The drawing under review shows one solid part. Ordinate dimensions are in mm from its lowest x, y, z. Coordinates: 2 decimals unless noted, no trailing zeros. Write each loop counter-clockwise with the first axis right and the second up, starting at its lowest first coordinate (ties: lowest second). Pieces come first, ordered by that corner, then holes. Notation, with made-up numbers: (26.5, 65) -> (45.5, 65) arc R21 ccw to (45.5, 81) -> close; hole circle Ø10 at (36, -18.75). An arc over 180 degrees is marked (long way). One line per question, with ' | ' between items. Start each with the question number.
Q1. Add section D-D on x = 3.5. State the section outline as (y, z) points, and give its area (3 significant figures).
Q2. Add section B-B on y = 1.8. State the section outline as (x, z) points, and give its area (3 significant figures).
Q3. Add section C-C on z = 61.5. State the section outline as (x, y) points, and give its area (3 significant figures).
Q4. Add section A-A on x = 26.5. State the section outline as (y, z) points, and give its area (3 significant figures).
Q5. Wall thickness on probe 1 along Z at (x, y) = (26.5, 1.9); probe 2 along Z at (x, y) = (3.5, 0.85); probe 3 along Z at (x, y) = (27, 2.1): over which ranges is each line inside the solid? List them lowest first.
Q6. For P1, Ø0.9, axis at y = 2, z = 24.5, coming from the +X side, flat-tipped, find the tip position at first contact; note if it passes through.
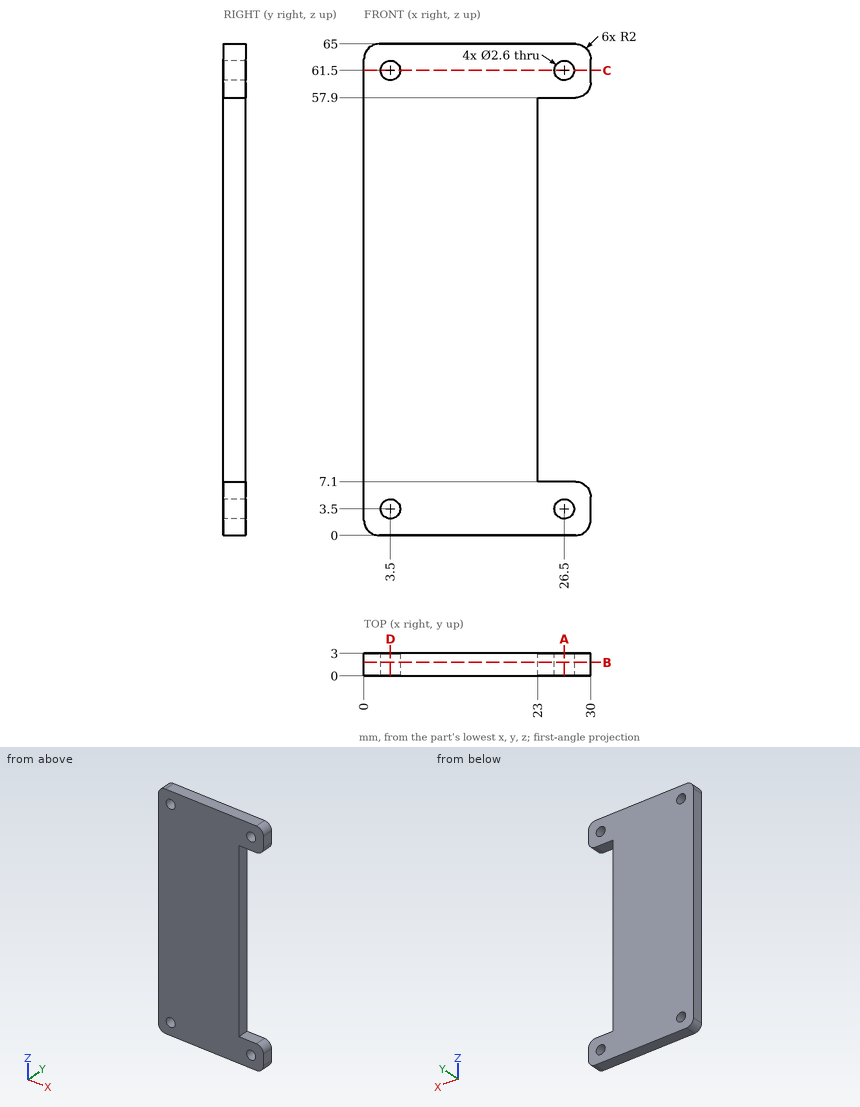
Output values:
1) outline: (0, 0) -> (3, 0) -> (3, 2.2) -> (0, 2.2) -> close; (0, 4.8) -> (3, 4.8) -> (3, 60.2) -> (0, 60.2) -> close; (0, 62.8) -> (3, 62.8) -> (3, 65) -> (0, 65) -> close | area: 179 mm2
2) outline: (0, 2) arc R2 ccw to (2, 0) -> (28, 0) arc R2 ccw to (30, 2) -> (30, 5.1) arc R2 ccw to (28, 7.1) -> (23, 7.1) -> (23, 57.9) -> (28, 57.9) arc R2 ccw to (30, 59.9) -> (30, 63) arc R2 ccw to (28, 65) -> (2, 65) arc R2 ccw to (0, 63) -> close; hole circle Ø2.6 at (3.5, 3.5); hole circle Ø2.6 at (3.5, 61.5); hole circle Ø2.6 at (26.5, 3.5); hole circle Ø2.6 at (26.5, 61.5) | area: 1,570 mm2
3) outline: (0, 0) -> (2.2, 0) -> (2.2, 3) -> (0, 3) -> close; (4.8, 0) -> (25.2, 0) -> (25.2, 3) -> (4.8, 3) -> close; (27.8, 0) -> (30, 0) -> (30, 3) -> (27.8, 3) -> close | area: 74.4 mm2
4) outline: (0, 0) -> (3, 0) -> (3, 2.2) -> (0, 2.2) -> close; (0, 4.8) -> (3, 4.8) -> (3, 7.1) -> (0, 7.1) -> close; (0, 57.9) -> (3, 57.9) -> (3, 60.2) -> (0, 60.2) -> close; (0, 62.8) -> (3, 62.8) -> (3, 65) -> (0, 65) -> close | area: 27.0 mm2
5) probe 1: z = 0 to 2.2, 4.8 to 7.1, 57.9 to 60.2, 62.8 to 65 | probe 2: z = 0 to 2.2, 4.8 to 60.2, 62.8 to 65 | probe 3: z = 0 to 2.3, 4.7 to 7.1, 57.9 to 60.3, 62.7 to 65
6) P1: stops at x = 23
